Could you check a few things on this model? Use its own coordinates, in mm. Face numbers are marked on the shaded views. A direction names the side the tool comes from. Give positions to 0.01 mm unless a question says otherwise; leave off trailing zeros. Write each loop counter-clockwise with the first axis right and the second up, starting at its lowest first coordinate (ties: lowest second). Pieces come first, ordered by that corner, then holes. Notation, with made-up numbers: (2, 89) - (24, 89) arc R18 ccw to (24, 124) - close; hole circle Ø6 at (18, 45.25). An arc over 180 degrees is marked (long way). Answer as CSV lines item,"result". Start each with the question number.
Q1. Imagine slicing it at B-B on x = 0. List the corners of the cut face in (y, z) for me (3 decimals), and give its area (4 significant figures).
Q2. Imagine slicing it at C-C on z = 0.75. List the corners of the cut face in (x, y) for me (3 decimals), and give its area (3 significant figures).
Q3. If I drill on line 1 along Y through (x, z) = (0, 6.25) (3 decimals); line 2 along Z through (x, y) = (-1.75, -2); line 3 along X through (y, z) = (-2, 5.25), over which ranges is the centre line in solid material (lowest first)?
Q4. We'd pull the mould along Y, two halves only. Please class the marked faces 3, 4 and 5: pulls with the +Y half, pulls with the -Y half, needs draft (parallel to the pull), parting line crosses it, or undercut.
Q5. On a 3-axis mill with a long thin cutter (end or side, diameter ignored), from which of +Z, -Z, +X, -X, +Y, -Y can I reach the whole of each face in a straight line? I mean the marked faces 1 and 2. Say none if no direction works.
Q6. Will these pins go through, and if not, where does the flat tip stop? pin 1 Ø2 at (y, z) = (1, 1.5) entering from -X; pin 2 Ø3 at (y, z) = (2, 1.5) entering from -X; pin 3 Ø0.6 at (y, z) = (4, 6.5) entering from -X.
Q7. Imagine slicing it at A-A on z = 3.75. List the corners of the cut face in (x, y) for me (3 decimals).
```python
from build123d import *

# Parameters (mm, degrees)
F0_R     = 5.625
F1_DEPTH = 8
F2_DEPTH = 2
F3_SIZE  = 2.5


with BuildPart() as f1:
    # F0 (on Top) → F1 (new body)
    with BuildSketch(Plane.XY):
        Circle(F0_R)
        with BuildLine():
            ThreePointArc((1, 3.48434), (2.895309, 2.181241), (3.625, 0))
            ThreePointArc((3.625, 0), (-2.181241, -2.895309), (-1, 3.48434))
            Line((-1, 3.48434), (-1, 4.625))
            Line((-1, 4.625), (1, 4.625))
            Line((1, 4.625), (1, 3.48434))
        make_face(mode=Mode.SUBTRACT)
    extrude(amount=F1_DEPTH)

    # F0 (on Top) → F2 (join)
    with BuildSketch(Plane.XY):
        with BuildLine():
            ThreePointArc((-1, 3.48434), (-2.181241, -2.895309), (3.625, 0))
            ThreePointArc((3.625, 0), (2.895309, 2.181241), (1, 3.48434))
            Line((1, 3.48434), (1, 2.625))
            Line((1, 2.625), (-1, 2.625))
            Line((-1, 2.625), (-1, 3.48434))
        make_face()
        with BuildLine():
            ThreePointArc((-1, 3.48434), (0, 3.625), (1, 3.48434))
            Line((1, 3.48434), (1, 4.625))
            Line((1, 4.625), (-1, 4.625))
            Line((-1, 4.625), (-1, 3.48434))
        make_face()
        with BuildLine():
            Line((1, 2.625), (1, 3.48434))
            ThreePointArc((1, 3.48434), (0, 3.625), (-1, 3.48434))
            Line((-1, 3.48434), (-1, 2.625))
            Line((-1, 2.625), (1, 2.625))
        make_face()
    extrude(amount=F2_DEPTH)

    # F3
    f3_edges = [f1.edges().sort_by_distance(p)[0] for p in [
        (-5.625, 0, 0),
    ]]
    chamfer(f3_edges, length=F3_SIZE)


solid = f1.part
```
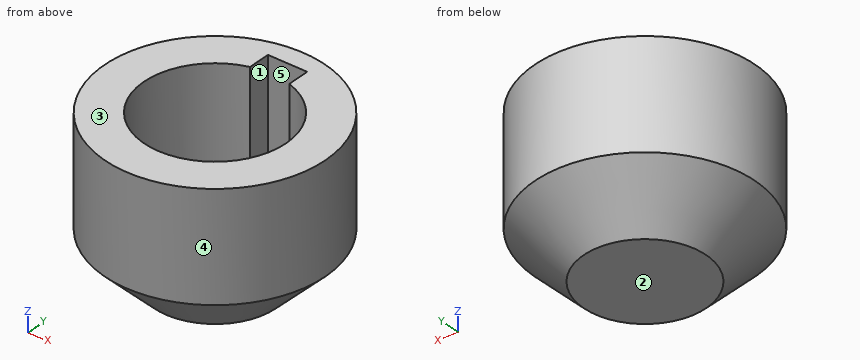
Conclusion:
1,outline,"(-5.625, 2.5) - (-3.125, 0) - (3.125, 0) - (5.625, 2.5) - (5.625, 8) - (4.625, 8) - (4.625, 2) - (-3.625, 2) - (-3.625, 8) - (-5.625, 8) - close"
1,area,"34.25 mm^2"
2,outline,"circle Ø7.75 at (0, 0)"
2,area,"47.2 mm^2"
3,line 1,"-5.625 to -3.625, 4.625 to 5.625"
3,line 2,"0 to 2"
3,line 3,"-5.26 to -3.02, 3.02 to 5.26"
4,face 3,"needs draft"
4,face 4,"parting line crosses it"
4,face 5,"undercut"
5,face 1,"+Z"
5,face 2,"-Z, +X, -X, +Y, -Y"
6,pin 1,"x = -5.55"
6,pin 2,"x = -5.56"
6,pin 3,"x = -4.24"
7,outline,"circle Ø11.25 at (0, 0); hole (-1, 3.484) arc R3.625 ccw (long way) to (1, 3.484) - (1, 4.625) - (-1, 4.625) - close"
